```python
from build123d import *

# Parameters (mm, degrees)
SKETCH1_W           = 79.9338
SKETCH1_H           = 36.0426
BOSS_EXTRUDE1_DEPTH = 1.6256
SKETCH2_W           = 70.993
SKETCH2_H           = 26.3144
BOSS_EXTRUDE2_DEPTH = 8.5344
SKETCH3_W           = 40.64
SKETCH3_H           = 2.54
BOSS_EXTRUDE3_DEPTH = 8.3312


with BuildPart() as part:
    # Sketch1 → Boss-Extrude1 (new body)
    with BuildSketch(Plane(origin=(0, 0, 0), x_dir=(1, 0, 0), z_dir=(0, 1, 0))):
        Rectangle(SKETCH1_W, SKETCH1_H)
    extrude(amount=BOSS_EXTRUDE1_DEPTH)

    # Sketch2 → Boss-Extrude2 (add)
    with BuildSketch(Plane(origin=(0, 1.6256, 0), x_dir=(1, 0, 0), z_dir=(0, 1, 0))):
        with Locations((0, -0.1143)):
            Rectangle(SKETCH2_W, SKETCH2_H)
    extrude(amount=BOSS_EXTRUDE2_DEPTH)

    # Sketch3 → Boss-Extrude3 (add)
    with BuildSketch(Plane.XZ):
        with Locations((-12.9159, -15.7099)):
            Rectangle(SKETCH3_W, SKETCH3_H)
    extrude(amount=BOSS_EXTRUDE3_DEPTH)


solid = part.part
```
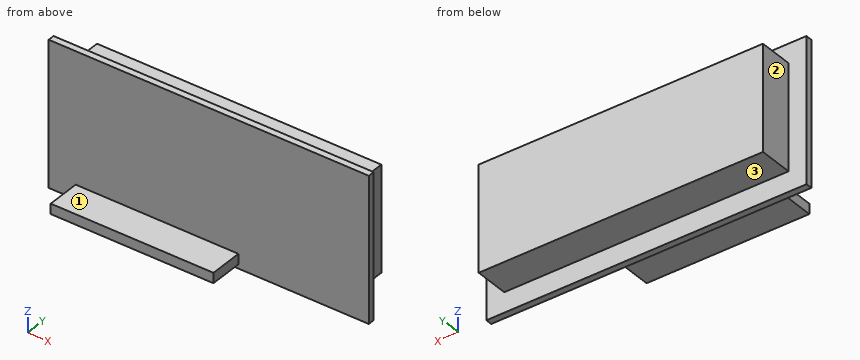
Input: part model. Units: mm. Frame: model coordinates. Face numbers are marked on the shaded views. A direction names the side the tool comes from. Round coordinates to 2 decimals unless told otherwise and drop trailing zeros. Loops run counter-clockwise (first coordinate to the right, second up) from the corner with the lowest first, then second, coordinate; pieces in that order, holes last.
1) Pin query (flat end, axial travel): pin 1 (2.5 mm diameter, centred on y = 5.5, z = -3.5, fed in from +X); pin 2 (4 mm diameter, centred on x = -9.5, y = -3, fed in from +Z); pin 3 (7 mm diameter, centred on y = 6, z = -4, fed in from -X). Return the tip coordinate at first contact, or that it passes through.
Ans:
pin 1: stops at x = 35.5
pin 2: stops at z = -14.44
pin 3: stops at x = -35.5
2) Section query B-B on x = -29. Return the cut outline in (y, z).
Ans:
outline: (-8.33, -16.98) - (0, -16.98) - (0, -18.02) - (1.63, -18.02) - (1.63, -13.04) - (10.16, -13.04) - (10.16, 13.27) - (1.63, 13.27) - (1.63, 18.02) - (0, 18.02) - (0, -14.44) - (-8.33, -14.44) - close
3) Section query C-C on y = 3. Return the cut outline in (x, z), plus the area to 3 significant figures.
Ans:
outline: (-35.5, -13.04) - (35.5, -13.04) - (35.5, 13.27) - (-35.5, 13.27) - close
area: 1,870 mm2
4) Set-up query: the marked faces 1, 2 and 3. Return all of +Z, -Z, +X, -X, +Y, -Y with unobstructed straight access to the full face (end or side cutting, diameter ignored); none if empty.
Ans:
face 1: +Z, +X, -X, -Y
face 2: +Z, -Z, -X, +Y
face 3: -Z, +X, -X, +Y
5) Section query A-A on z = 3. Return the cut outline in (x, y).
Ans:
outline: (-39.97, 0) - (39.97, 0) - (39.97, 1.63) - (35.5, 1.63) - (35.5, 10.16) - (-35.5, 10.16) - (-35.5, 1.63) - (-39.97, 1.63) - close
6) Material intervals for line 1 (X direction, y = 9, z = -6.5); line 2 (Y direction, x = 5, z = 5); line 3 (Z direction, x = -18.5, y = 1.75), sorted ascending.
Ans:
line 1: x = -35.5 to 35.5
line 2: y = 0 to 10.16
line 3: z = -13.04 to 13.27
7) Section query D-D on x = 11.5. Return the cut outline in (y, z).
Ans:
outline: (0, -18.02) - (1.63, -18.02) - (1.63, -13.04) - (10.16, -13.04) - (10.16, 13.27) - (1.63, 13.27) - (1.63, 18.02) - (0, 18.02) - close
